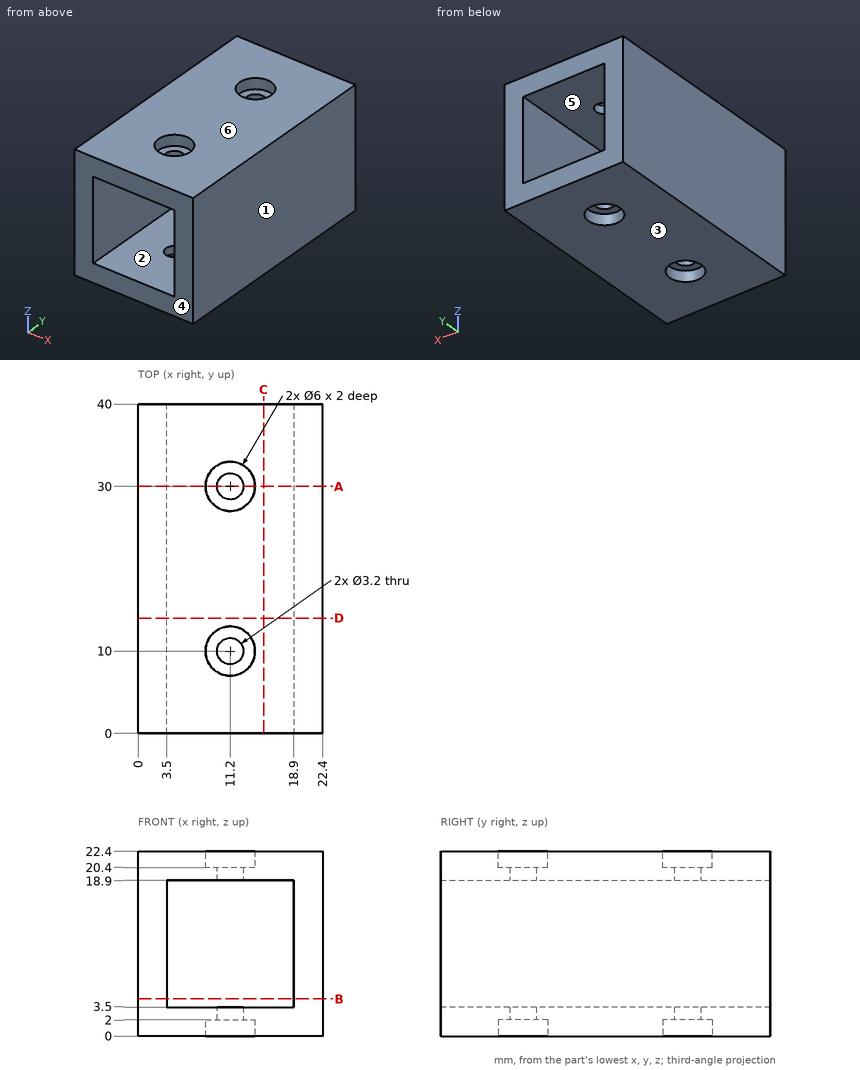
The figure shows three views and two pictorial views of one solid part (mm, origin at its lowest corner). Answer the questions. A direction names the side the tool comes from. Round coordinates to 2 decimals unless told otherwise and drop trailing zeros. Loops run counter-clockwise (first coordinate to the right, second up) from the corner with the lowest first, then second, coordinate; pieces in that order, holes last. Notation, with made-up numbers: (42.25, 1) - (81.25, 1) arc R34 ccw to (81.25, 38) - close; hole circle Ø10 at (24.25, 76). An arc over 180 degrees is marked (long way). Use one line per item in the form item = value. Start each with the question number.
(1) Find section A-A on y = 30. Determine the outline of the cut face in (x, z).
(2) Flat-ended cylindrical pins translate along their axes: P1, Ø1.5, axis at x = 11.5, y = 21, coming from the -Z side; P2, Ø3.5, axis at x = 11.2, y = 30, coming from the +Z side; P3, Ø3.5, axis at x = 11.2, y = 10, coming from the -Z side. Find the tip coordinate at first contact, or state that the pin passes through.
(3) Find section C-C on x = 15.25. Determine the outline of the cut face in (y, z), and give its area (3 significant figures).
(4) Determine the mould class of the marked faces 3, 4, 5 and 6 for opening direction Z: +Z half, -Z half, draft (parallel to the pull), parting line (faces both ways), or undercut.
(5) Consider line 1 (Y direction, x = 11.2, z = 20.9); line 2 (Y direction, x = 11.2, z = 2.45); line 3 (Z direction, x = 13.75, y = 18.5). Determine where each line is inside the solid, lowest interval first.
(6) Find section D-D on y = 14. Determine the outline of the cut face in (x, z), and give its area (3 significant figures).
(7) Which of the six approach directions +Z, -Z, +X, -X, +Y, -Y give full straight-line access (tool end or side, diameter ignored) to the marked faces 1 and 2?
(8) Find section B-B on z = 4.5. Determine the outline of the cut face in (x, y).
Answer list:
q1.outline = (0, 0) - (8.2, 0) - (8.2, 2) - (9.6, 2) - (9.6, 3.5) - (3.5, 3.5) - (3.5, 18.9) - (9.6, 18.9) - (9.6, 20.4) - (8.2, 20.4) - (8.2, 22.4) - (0, 22.4) - close; (12.8, 2) - (14.2, 2) - (14.2, 0) - (22.4, 0) - (22.4, 22.4) - (14.2, 22.4) - (14.2, 20.4) - (12.8, 20.4) - (12.8, 18.9) - (18.9, 18.9) - (18.9, 3.5) - (12.8, 3.5) - close
q2.P1 = 0
q2.P2 = 20.4
q2.P3 = 2
q3.outline = (0, 0) - (40, 0) - (40, 3.5) - (0, 3.5) - close; (0, 18.9) - (40, 18.9) - (40, 22.4) - (0, 22.4) - close
q3.area = 280 mm^2
q4.face_3 = -Z half
q4.face_4 = draft
q4.face_5 = undercut
q4.face_6 = +Z half
q5.line_1 = 0 to 7, 13 to 27, 33 to 40
q5.line_2 = 0 to 8.4, 11.6 to 28.4, 31.6 to 40
q5.line_3 = 0 to 3.5, 18.9 to 22.4
q6.outline = (0, 0) - (22.4, 0) - (22.4, 22.4) - (0, 22.4) - close; hole (3.5, 3.5) - (18.9, 3.5) - (18.9, 18.9) - (3.5, 18.9) - close
q6.area = 265 mm^2
q7.face_1 = +Z, -Z, +X, +Y, -Y
q7.face_2 = +Y, -Y
q8.outline = (0, 0) - (3.5, 0) - (3.5, 40) - (0, 40) - close; (18.9, 0) - (22.4, 0) - (22.4, 40) - (18.9, 40) - close
